The listing builds one solid part. Answer for the finished solid, in the listing's coordinates (mm). Face numbers are marked on the shaded views. A direction names the side the tool comes from. Round coordinates to 2 decimals unless told otherwise and drop trailing zeros. Loops run counter-clockwise (first coordinate to the right, second up) from the corner with the lowest first, then second, coordinate; pieces in that order, holes last. Notation, with made-up numbers: (77, 78.5) -> (133, 78.5) arc R10 ccw to (133, 92.5) -> close; hole circle Ø1 at (47, 22.5). An arc over 180 degrees is marked (long way). Answer in a Markdown table with one row per item. Add a question column.
```python
from build123d import *

# Parameters (mm, degrees)
BOSS_EXTRUDE1_DEPTH = 22.86
BOSS_EXTRUDE2_DEPTH = 13.462
BOSS_EXTRUDE3_START = -1.27
BOSS_EXTRUDE3_DEPTH = 1.905
BOSS_EXTRUDE4_START = -1.27
BOSS_EXTRUDE4_DEPTH = 3.81
SKETCH8_R           = 2.8
SKETCH8_R_2         = 1.5875
CUT_EXTRUDE1_DEPTH  = 8
SKETCH9_W           = 28.575
SKETCH9_H           = 11.43
CUT_EXTRUDE2_DEPTH  = 13.7
FILLET1_R           = 1.27


with BuildPart() as part:
    # Sketch1 → Boss-Extrude1 (new body)
    with BuildSketch(Plane.XY):
        Polygon((-6.096, 10.16), (6.096, 10.16), (6.096, 0), (14.2875, 0), (14.2875, 6.35), (8.636, 7.346511931), (8.636, 12.7), (-8.636, 12.7), (-8.636, 7.346511931), (-14.2875, 6.35), (-14.2875, 0), (-6.096, 0), align=None)
    extrude(amount=-BOSS_EXTRUDE1_DEPTH)

    # Sketch2 → Boss-Extrude2 (add)
    with BuildSketch(Plane.XY):
        with BuildLine():
            Line((2.921, 10.16), (6.096, 10.16))
            Line((6.096, 10.16), (6.096, 6.985))
            ThreePointArc((6.096, 6.985), (5.16606403, 9.23006403), (2.921, 10.16))
        make_face()
        with BuildLine():
            Line((-6.096, 10.16), (-6.096, 6.985))
            ThreePointArc((-6.096, 6.985), (-5.16606403, 9.23006403), (-2.921, 10.16))
            Line((-2.921, 10.16), (-6.096, 10.16))
        make_face()
    extrude(amount=-BOSS_EXTRUDE2_DEPTH)

    # Sketch3 → Boss-Extrude3 (add)
    with BuildSketch(Plane.XY.offset(-13.462).offset(BOSS_EXTRUDE3_START)):
        with BuildLine():
            Line((-6.096, 10.16), (-6.096, 6.985))
            ThreePointArc((-6.096, 6.985), (-5.16606403, 9.23006403), (-2.921, 10.16))
            Line((-2.921, 10.16), (-6.096, 10.16))
        make_face()
    extrude(amount=-BOSS_EXTRUDE3_DEPTH)

    # Sketch4 → Boss-Extrude4 (add)
    with BuildSketch(Plane.XY.offset(-16.637).offset(BOSS_EXTRUDE4_START)):
        with BuildLine():
            Line((-6.096, 10.16), (-6.096, 6.985))
            ThreePointArc((-6.096, 6.985), (-5.16606403, 9.23006403), (-2.921, 10.16))
            Line((-2.921, 10.16), (-6.096, 10.16))
        make_face()
    extrude(amount=-BOSS_EXTRUDE4_DEPTH)

    # Sketch6 → Cut-Revolve1 (revolve, cut)
    with BuildSketch(Plane.XY.offset(-5.08)):
        Polygon((11.262482277, -1.27), (12.849982277, -1.27), (12.849982277, 6.60347316), (12.849982277, 9.423392242), (11.262482277, 9.423392242), (11.262482277, 6.883392242), align=None)
    cut_revolve1 = revolve(axis=Axis((11.262482277, -1.27, -5.08), (0, -1, 0)), mode=Mode.SUBTRACT)

    # Mirror1: Cut-Revolve1 across plane
    add(cut_revolve1.mirror(Plane(origin=(0, 0, 0), x_dir=(0, 0, 1), z_dir=(1, 0, 0))), mode=Mode.SUBTRACT)

    # Mirror2: Cut-Revolve1 across plane
    add(cut_revolve1.mirror(Plane.XY.offset(-11.43)), mode=Mode.SUBTRACT)

    # Mirror2 copy 1 sketch → Mirror2 copy 1 (revolve, cut)
    with BuildSketch(Plane(origin=(0, 0, -17.78), x_dir=(-1, 0, 0), z_dir=(0, 0, -1))):
        Polygon((11.262482277, -1.27), (12.849982277, -1.27), (12.849982277, 6.60347316), (12.849982277, 9.423392242), (11.262482277, 9.423392242), (11.262482277, 6.883392242), align=None)
    revolve(axis=Axis((-11.262482277, -1.27, -17.78), (0, -1, 0)), mode=Mode.SUBTRACT)

    # Sketch8 → Cut-Extrude1 (cut)
    with BuildSketch(Plane(origin=(0, 12.7, 0), x_dir=(-1, 0, 0), z_dir=(0, -1, 0))):
        with Locations((11.262482277, 17.78)):
            Circle(SKETCH8_R)
        with Locations((11.262482277, 17.78)):
            Circle(SKETCH8_R_2, mode=Mode.SUBTRACT)
        with Locations((11.262482277, 5.08)):
            Circle(SKETCH8_R)
        with Locations((11.262482277, 5.08)):
            Circle(SKETCH8_R_2, mode=Mode.SUBTRACT)
        with Locations((-11.262482277, 5.08)):
            Circle(SKETCH8_R)
        with Locations((-11.262482277, 5.08)):
            Circle(SKETCH8_R_2, mode=Mode.SUBTRACT)
        with Locations((-11.262482277, 17.78)):
            Circle(SKETCH8_R)
        with Locations((-11.262482277, 17.78)):
            Circle(SKETCH8_R_2, mode=Mode.SUBTRACT)
    extrude(amount=CUT_EXTRUDE1_DEPTH, mode=Mode.SUBTRACT)

    # Sketch9 → Cut-Extrude2 (cut, through all)
    with BuildSketch(Plane(origin=(0, 0, 0), x_dir=(-1, 0, 0), z_dir=(0, -1, 0))):
        with Locations((0, 5.715)):
            Rectangle(SKETCH9_W, SKETCH9_H)
    extrude(amount=-CUT_EXTRUDE2_DEPTH, mode=Mode.SUBTRACT)

    # Fillet1
    fillet1_edges = [part.edges().sort_by_distance(p)[0] for p in [
        (-14.2875, 3.175, -22.86),
        (14.2875, 3.175, -22.86),
        (-8.636, 7.346511931, -14.119821979),
        (-8.636, 7.346511931, -20.805178021),
        (8.636, 7.346511931, -20.805178021),
        (8.636, 7.346511931, -14.119821979),
        (14.2875, 3.175, -11.43),
        (-14.2875, 3.175, -11.43),
    ]]
    fillet(fillet1_edges, radius=FILLET1_R)


solid = part.part
```
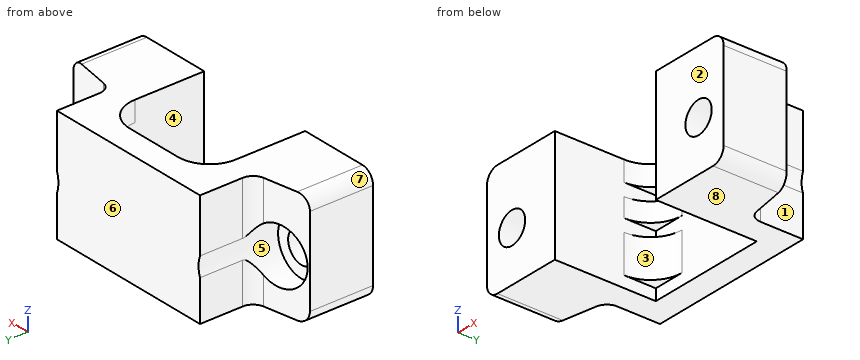
Item 1: Consider L1, parallel to X at y = 1.6, z = -17.78; L2, parallel to X at y = 3.25, z = -15.25; L3, parallel to X at y = 3, z = -17. Determine where each line is inside the solid, lowest interval first. Write a range as from..to.
Item 2: Section B-B, the plane y = 8 is taken. Write down the section's boundary in (x, z).
Item 3: Section C-C, the plane y = 3.25 is taken. Write down the section's boundary in (x, z) (1 decimal).
Item 4: For the marked faces 1, 2, 3 and 4, determine the directions among +Z, -Z, +X, -X, +Y, -Y from which every point of the face is accessible in a straight line to the end or side of a thin tool.
Item 5: Section A-A, the plane y = 5.5 is taken. Write down the section's boundary in (x, z), and give its area (3 significant figures).
Item 6: Flat-ended cylindrical pins translate along their axes: P1, Ø1.7, axis at x = 12, z = -18.5, coming from the +Y side; P2, Ø3.5, axis at y = 9.5, z = -20, coming from the +X side; P3, Ø4, axis at y = 11.5, z = -19.5, coming from the +X side. Find the tip coordinate at first contact, or state that the pin passes through.
Item 7: The mould has two halves that part along Z. Classify the marked faces 5, 6, 7 and 8: +Z half, -Z half, draft (parallel to the pull), parting line (faces both ways), or undercut.
Item 8: Section D-D, the plane x = 9.25 is taken. Write down the section's boundary in (y, z), and give its area (3 significant figures).
Here are the results:
| question | item | result |
|---|---|---|
| 1 | L1 | x = -14.29..-12.85, -9.67..-6.1, 6.1..9.67, 12.85..14.29 |
| 1 | L2 | x = -14.29..-6.1, 6.1..14.29 |
| 1 | L3 | x = -14.29..-12.65, -9.88..-6.1, 6.1..9.88, 12.65..14.29 |
| 2 | outline | (-8.7, -22.86) -> (-6.1, -22.86) -> (-6.1, -21.72) -> (-5.93, -21.72) -> (-5.93, -17.91) -> (-6.1, -17.91) -> (-6.1, -16.64) -> (-5.93, -16.64) -> (-5.93, -14.73) -> (-6.1, -14.73) -> (-6.1, -13.46) -> (-5.93, -13.46) -> (-5.93, -11.43) -> (-8.7, -11.43) -> (-8.7, -16.64) arc R2.8 cw to (-8.7, -18.92) -> close; (5.93, -13.46) -> (6.1, -13.46) -> (6.1, -22.86) -> (8.7, -22.86) -> (8.7, -18.92) arc R2.8 cw to (8.7, -16.64) -> (8.7, -11.43) -> (5.93, -11.43) -> close |
| 3 | outline | (-14.3, -21.6) arc R1.3 ccw to (-13, -22.9) -> (-6.1, -22.9) -> (-6.1, -11.4) -> (-13, -11.4) arc R1.3 ccw to (-14.3, -12.7) -> close; (6.1, -22.9) -> (13, -22.9) arc R1.3 ccw to (14.3, -21.6) -> (14.3, -12.7) arc R1.3 ccw to (13, -11.4) -> (6.1, -11.4) -> close; hole circle Ø3.2 at (-11.3, -17.8); hole circle Ø3.2 at (11.3, -17.8) |
| 4 | face 1 | +Z, -Z, +X, +Y |
| 4 | face 2 | +Z, -Z, +X, -X, -Y |
| 4 | face 3 | +Z, -Z, -Y |
| 4 | face 4 | -Z, -Y |
| 5 | outline | (-14.29, -21.59) arc R1.27 ccw to (-13.02, -22.86) -> (-6.1, -22.86) -> (-6.1, -11.43) -> (-13.02, -11.43) arc R1.27 ccw to (-14.29, -12.7) -> close; (6.1, -22.86) -> (13.02, -22.86) arc R1.27 ccw to (14.29, -21.59) -> (14.29, -12.7) arc R1.27 ccw to (13.02, -11.43) -> (6.1, -11.43) -> close; hole circle Ø5.6 at (-11.26, -17.78); hole circle Ø5.6 at (11.26, -17.78) |
| 5 | area | 137 mm² |
| 6 | P1 | stops at y = 4.7 |
| 6 | P2 | stops at x = 8.82 |
| 6 | P3 | stops at x = 8.64 |
| 7 | face 5 | undercut |
| 7 | face 6 | draft |
| 7 | face 7 | +Z half |
| 7 | face 8 | -Z half |
| 8 | outline | (0, -22.86) -> (7.32, -22.86) -> (7.32, -19.73) -> (4.7, -19.73) -> (4.7, -15.83) -> (7.32, -15.83) -> (7.32, -11.43) -> (0, -11.43) -> close |
| 8 | area | 73.5 mm² |
